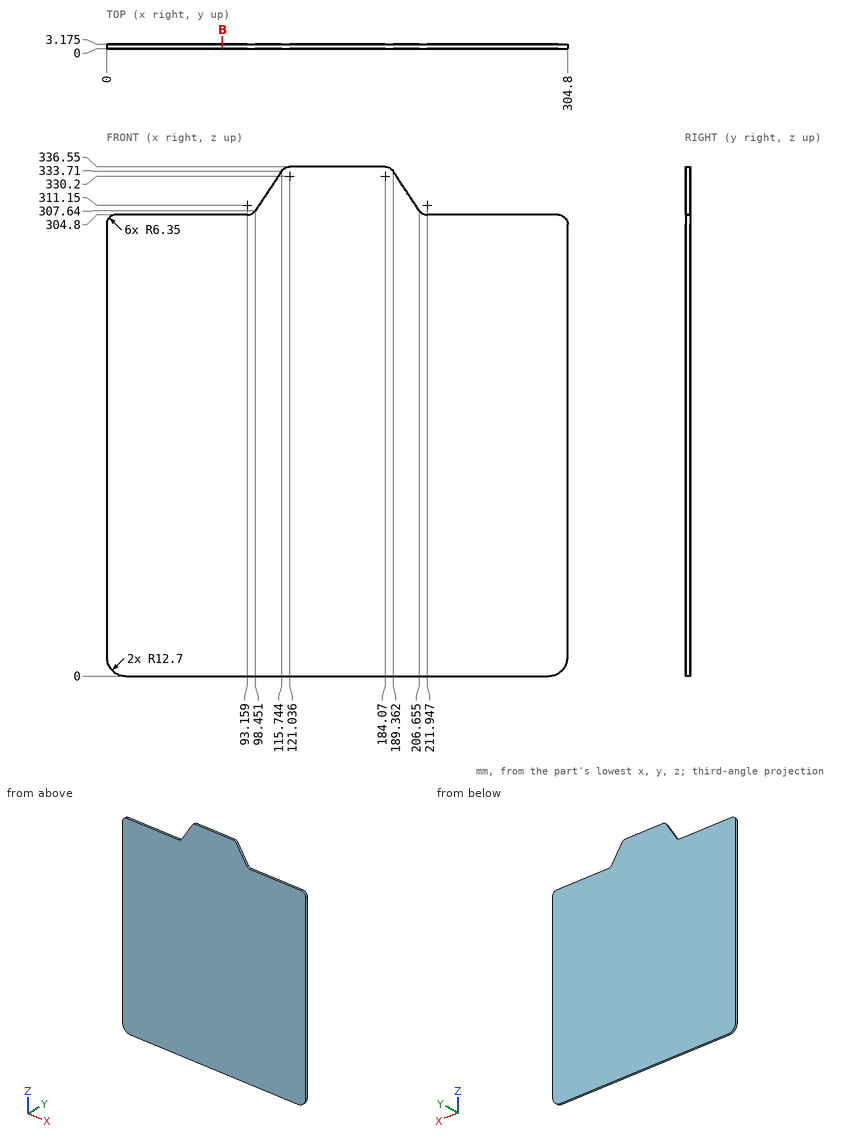
Design review of the part shown in the three views and the two pictorial views. Dimensions are in mm from the part's minimum x, y and z. Give positions to 0.01 mm unless a question says otherwise; leave off trailing zeros. Write each loop counter-clockwise with the first axis right and the second up, starting at its lowest first coordinate (ties: lowest second). Pieces come first, ordered by that corner, then holes. Notation, with made-up numbers: (59.25, 19) -> (85.25, 19) arc R15 ccw to (85.25, 45) -> close; hole circle Ø5 at (47, 65). An arc over 180 degrees is marked (long way). Answer in a Markdown table with one row per item.
1) Add section B-B on x = 76.5. State the section outline as (y, z) points (1 decimal).
Worked answers:
| item | result |
|---|---|
| outline | (0, 0) -> (3.2, 0) -> (3.2, 304.8) -> (0, 304.8) -> close |
2) Clearance check with flat-ended pins moving along their axes: P1, Ø1, axis at x = 34.5, y = 1, coming from the +Z side; P2, Ø1, axis at x = 118, y = 2.5, coming from the +Z side. State where each tip first meets the part, or that it passes through.
Worked answers:
| item | result |
|---|---|
| P1 | z = 304.8 |
| P2 | z = 336.02 |
3) For L1, parallel to Z at x = 89, y = 2.85; L2, parallel to X at y = 2, z = 303.5; L3, parallel to Z at x = 209.5, y = 1.2, list the stretches that pass through material, from the lowest coordinate up. Write a range as [from, to].
Worked answers:
| item | result |
|---|---|
| L1 | [0, 304.8] |
| L2 | [2.5, 302.3] |
| L3 | [0, 305.29] |
